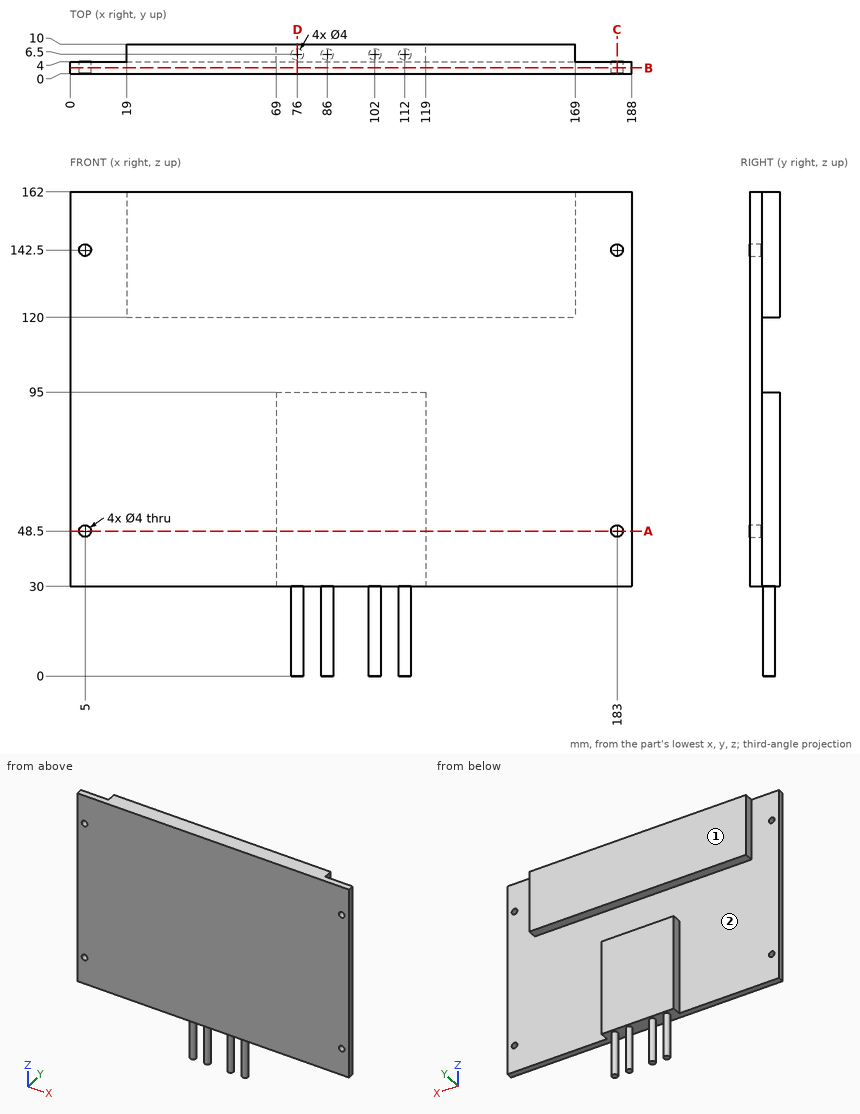
Answer from the drawing. Dimensions are ordinates in mm from the lowest x, y and z of the part. Round coordinates to 2 decimals unless told otherwise and drop trailing zeros. Write each loop counter-clockwise with the first axis right and the second up, starting at its lowest first coordinate (ties: lowest second). Pieces come first, ordered by that corner, then holes. Notation, with made-up numbers: (88, 55) -> (110, 55) arc R31 ccw to (110, 88) -> close; hole circle Ø11 at (70.5, 39.25). An arc over 180 degrees is marked (long way). Answer in a Markdown table with one row per item. Add a question column.
1) Find section B-B, the plane y = 2. Determine the outline of the cut face in (x, z).
2) Find section C-C, the plane x = 183. Determine the outline of the cut face in (y, z).
3) Determine the mould class of the marked faces 1 and 2 for opening direction Z: pulls with the +Z half, pulls with the -Z half, needs draft (parallel to the pull), parting line crosses it, or undercut.
4) Find section A-A, the plane z = 48.5. Determine the outline of the cut face in (x, y), and give its area (3 significant figures).
5) Given P1, Ø4.5, axis at x = 183, z = 48.5, coming from the -Y side; P2, Ø1.8, axis at y = 8, z = 51.5, coming from the +X side; P3, Ø2.5, axis at x = 183, z = 142.5, coming from the +Y side; P4, Ø1, axis at x = 161, z = 33, coming from the +Y side, each flat-ended and moving along its own axis, determine where each tip first touches the part or whether it passes through.
6) Find section D-D, the plane x = 76. Determine the outline of the cut face in (y, z), and give its area (3 significant figures).
7) Consider line 1 (X direction, y = 3.1, z = 48.5); line 2 (Z direction, x = 112, y = 5.5); line 3 (Z direction, x = 89, y = 9.75). Determine where each line is inside the solid, lowest interval first.
Findings below:
| question | item | result |
|---|---|---|
| 1 | outline | (0, 30) -> (188, 30) -> (188, 162) -> (0, 162) -> close; hole circle Ø4 at (5, 48.5); hole circle Ø4 at (5, 142.5); hole circle Ø4 at (183, 48.5); hole circle Ø4 at (183, 142.5) |
| 2 | outline | (0, 30) -> (4, 30) -> (4, 46.5) -> (0, 46.5) -> close; (0, 50.5) -> (4, 50.5) -> (4, 140.5) -> (0, 140.5) -> close; (0, 144.5) -> (4, 144.5) -> (4, 162) -> (0, 162) -> close |
| 3 | face 1 | needs draft |
| 3 | face 2 | undercut |
| 4 | outline | (0, 0) -> (3, 0) -> (3, 4) -> (0, 4) -> close; (7, 0) -> (181, 0) -> (181, 4) -> (119, 4) -> (119, 10) -> (69, 10) -> (69, 4) -> (7, 4) -> close; (185, 0) -> (188, 0) -> (188, 4) -> (185, 4) -> close |
| 4 | area | 1,020 mm² |
| 5 | P1 | y = 0 |
| 5 | P2 | x = 119 |
| 5 | P3 | through |
| 5 | P4 | y = 4 |
| 6 | outline | (0, 30) -> (4.5, 30) -> (4.5, 0) -> (8.5, 0) -> (8.5, 30) -> (10, 30) -> (10, 95) -> (4, 95) -> (4, 120) -> (10, 120) -> (10, 162) -> (0, 162) -> close |
| 6 | area | 1,290 mm² |
| 7 | line 1 | 0 to 3, 7 to 181, 185 to 188 |
| 7 | line 2 | 0 to 95, 120 to 162 |
| 7 | line 3 | 30 to 95, 120 to 162 |
